Part print with two shaded views. Sizes in mm from the minimum x, y, z corner. A direction names the side the tool comes from. Coordinates: 2 decimals unless noted, no trailing zeros. Order: outer loops, then holes, each group sorted by start corner. A loop starts at its lowest first (then second) coordinate and runs counter-clockwise, first axis right, second up. Notation, with made-up numbers: (76.5, 69.5) - (129.5, 69.5) arc R20 cw to (129.5, 108.5) - close; hole circle Ø1 at (-32, 46). An arc over 180 degrees is marked (long way). Write each question's results on one line, items separated by ' | '. Start each with the question number.
Q1. Wall check: probe 1 along Y at (x, z) = (8.5, 15.5); probe 2 along X at (y, z) = (22, 8.5) (1 decimal); probe 3 along Z at (x, y) = (17.5, 4.5) (1 decimal). Give the ranges that are in metal, low to high.
Q2. Pin check, flat tips, straight feed: P1, Ø1, axis at x = 5.5, y = 11, coming from the +Z side; P2, Ø5, axis at x = 8.5, y = 14, coming from the -Z side; P3, Ø3, axis at y = 40.5, z = 14, coming from the -X side (1 decimal). Stop position of each tip, or through.
Q3. Band-saw the part on B-B, the plane y = 10.5. Write the cut outline in (x, z) (1 decimal).
Q4. Band-saw the part on A-A, the plane x = 2.75. Write the cut outline in (y, z).
Q5. Which spindle directions (+Z, -Z, +X, -X, +Y, -Y) get a long thin tool onto all of the face, cutting with end or side? Do the marked faces 1 and 2. Say none if no direction does.
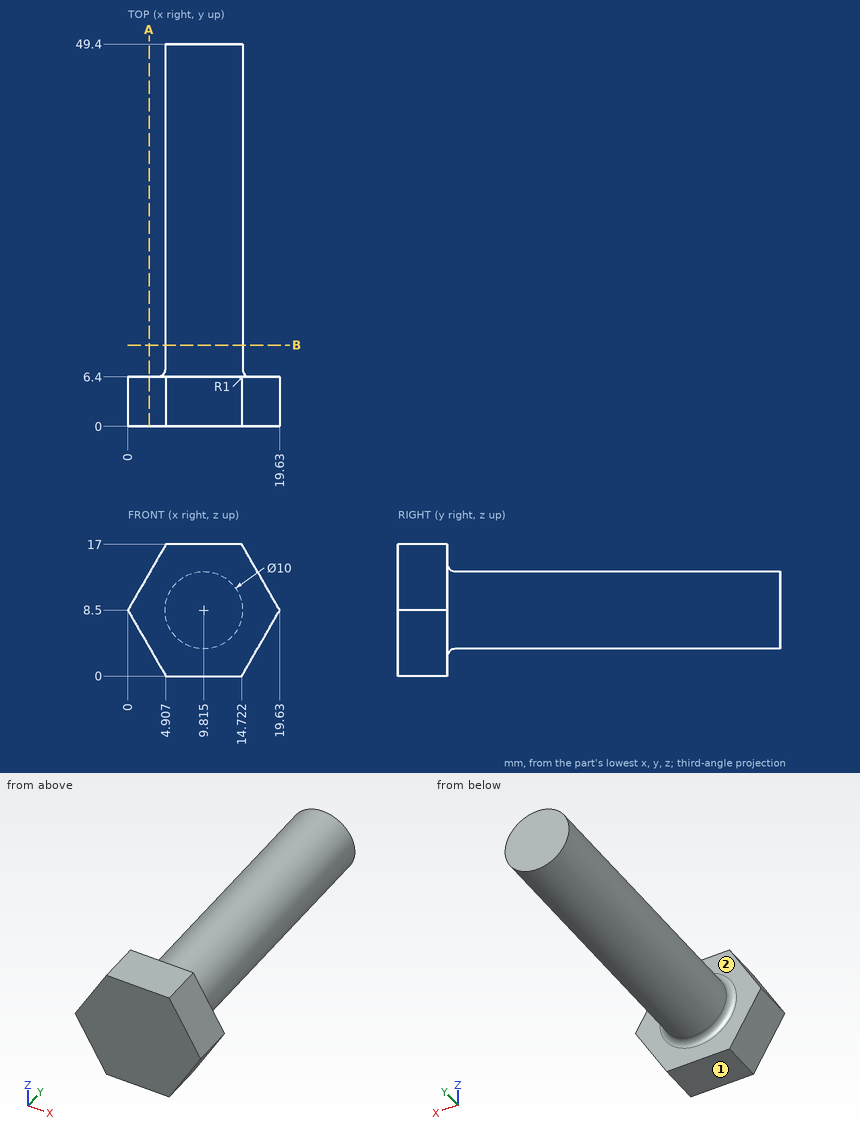
Results below:
1) probe 1: y = 0 to 6.4 | probe 2: x = 4.8 to 14.8 | probe 3: z = 4.8 to 12.2
2) P1: stops at z = 11.73 | P2: stops at z = 3.5 | P3: stops at x = 6.8
3) outline: circle Ø10 at (9.8, 8.5)
4) outline: (0, 3.74) - (6.4, 3.74) - (6.4, 13.26) - (0, 13.26) - close
5) face 1: -Z, +X, -X, +Y, -Y | face 2: +Y
